from build123d import *

# Parameters (mm, degrees)
SKETCH1_W           = 6
SKETCH1_H           = 70
SKETCH2_W           = 13
SKETCH2_H           = 13
BOSS_EXTRUDE1_DEPTH = 12


with BuildPart() as part:
    # Sketch1 → Revolve1 (revolve)
    with BuildSketch(Plane(origin=(0, 0, 0), x_dir=(1, 0, 0), z_dir=(0, 1, 0)), mode=Mode.PRIVATE) as revolve1_sk:
        with Locations((3, 35)):
            Rectangle(SKETCH1_W, SKETCH1_H)
    revolve(revolve1_sk.sketch.rotate(Axis((0, 0, -75.213634587), (0, 0, 1)), 180), axis=Axis((0, 0, -75.213634587), (0, 0, 1)))

    # Sketch2 → Boss-Extrude1 (add)
    with BuildSketch(Plane.XY.offset(-14)):
        Rectangle(SKETCH2_W, SKETCH2_H)
    extrude(amount=-BOSS_EXTRUDE1_DEPTH)


solid = part.part
Build history of the part. All positions in model axes, mm. A direction names the side the tool comes from. Coordinates: 2 decimals unless noted, no trailing zeros. Order: outer loops, then holes, each group sorted by start corner. A loop starts at its lowest first (then second) coordinate and runs counter-clockwise, first axis right, second up. Notation, with made-up numbers: (36, 36) - (52, 36) arc R13 cw to (52, 59) - close; hole circle Ø9 at (-38.5, 12.5). An arc over 180 degrees is marked (long way). Write item = value, one per line. Start each with the question number.
1) Flat gauge pins, fed straight in: pin 1 Ø1.5 at (y, z) = (1, -7) entering from +X; pin 2 Ø3 at (y, z) = (5, -48.5) entering from -X. Where does each tip first touch, or does it go through?
2) Wall check: line 1 along Z through (x, y) = (-5.5, 5.25); line 2 along X through (y, z) = (0.25, -6); line 3 along X through (y, z) = (-3.5, -58). Give the ranges that are in metal, low to high. Write a range as from..to.
3) 3-axis set-ups, long thin cutter, end or side, ignore diameter. For faces 1 (the face through (-4.4, -4.3, -26)), 2 (the face through (-5.723, -1.802, -7.098)), 3 (the face through (6.5, 0, -20)): which of +Z, -Z, +X, -X, +Y, -Y reach the whole face in a straight line?
4) Saw through at A-A on x = 0. Write the cut outline in (y, z), then the cut area to 3 significant figures.
5) Saw through at C-C on z = -36.5. Write the cut outline in (x, y).
From the geometry:
q1.pin_1 = 5.99
q1.pin_2 = -4.87
q2.line_1 = -26..-14
q2.line_2 = -5.99..5.99
q2.line_3 = -4.87..4.87
q3.face_1 = -Z
q3.face_2 = +Z
q3.face_3 = +Z, -Z, +X, +Y, -Y
q4.outline = (-6.5, -26) - (-6, -26) - (-6, -70) - (6, -70) - (6, -26) - (6.5, -26) - (6.5, -14) - (6, -14) - (6, 0) - (-6, 0) - (-6, -14) - (-6.5, -14) - close
q4.area = 852 mm^2
q5.outline = circle Ø12 at (0, 0)
